Print and shaded views of the part. All mm, measured from the part's lowest x, y and z. Coordinates: 2 decimals unless noted, no trailing zeros. Loops run counter-clockwise (first coordinate to the right, second up) from the corner with the lowest first, then second, coordinate; pieces in that order, holes last. Notation, with made-up numbers: M 49.25,63.25 L 103.25,63.25 A24 cw 103.25,91.25 Z; hole C 52.25,31.5 d6. An arc over 180 degrees is marked long. Answer as CSV lines item,"result". Start each with the question number.
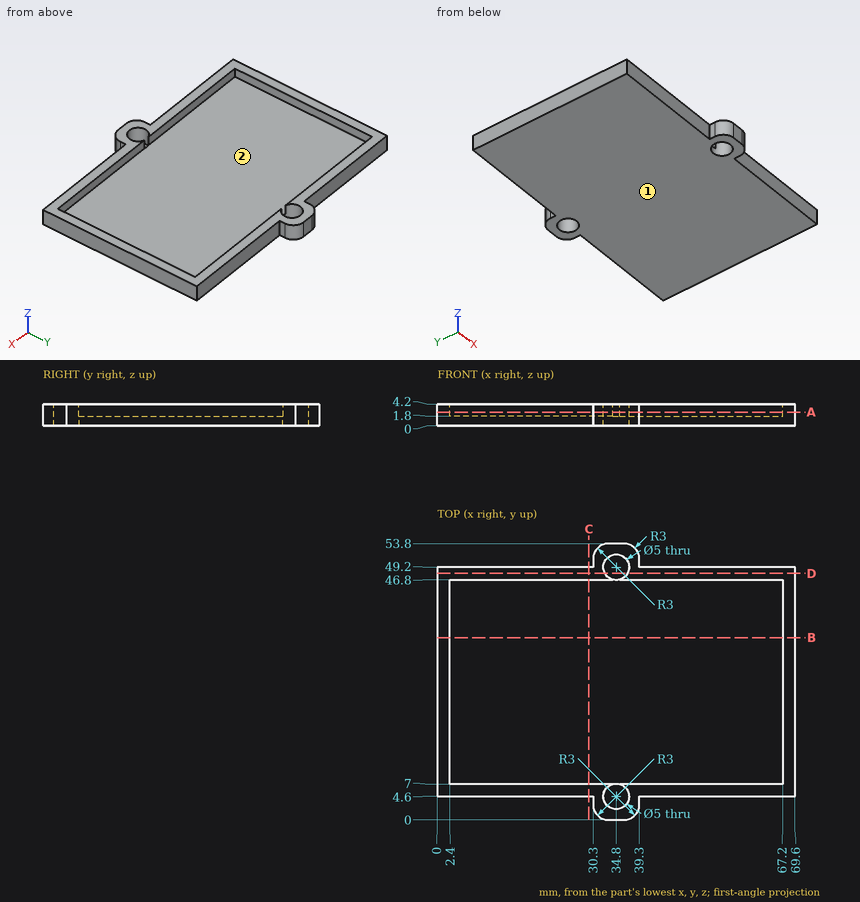
Q1. Flat gauge pins, fed straight in: P1, Ø1.3, axis at x = 22, z = 2, coming from the -Y side; P2, Ø0.8, axis at y = 50, z = 2, coming from the +X side; P3, Ø2, axis at x = 28.5, z = 0.5, coming from the +Y side. Where does each tip first touch, or does it go through?
Q2. Slice it at A-A, the plane z = 2.6. Write the cut outline in (x, y), and give its area (3 significant figures).
Q3. Slice it at C-C, the plane x = 29.5. Write the cut outline in (y, z), and give its area (3 significant figures).
Q4. Slice it at D-D, the plane y = 48. Write the cut outline in (x, z), and give its area (3 significant figures).
Q5. Slice it at B-B, the plane y = 35.5. Write the cut outline in (x, z).
Q6. Two-plate mould, pull along X, no slides. Class the marked faces 1 and 2: +X half, -X half, draft (parallel to the pull), parting line (faces both ways), or undercut.
Q7. Wall check: L1, parallel to Y at x = 34.8, z = 1.5; L2, parallel to Y at x = 43.5, z = 3.6; L3, parallel to X at y = 18.5, z = 3.1. Give the ranges that are in metal, low to high.
Solved:
1,P1,"stops at y = 4.6"
1,P2,"stops at x = 39.3"
1,P3,"stops at y = 49.2"
2,outline,"M 0,4.6 L 30.3,4.6 L 30.3,3 A3 ccw 33.3,0 L 36.3,0 A3 ccw 39.3,3 L 39.3,4.6 L 69.6,4.6 L 69.6,49.2 L 39.3,49.2 L 39.3,50.8 A3 ccw 36.3,53.8 L 33.3,53.8 A3 ccw 30.3,50.8 L 30.3,49.2 L 0,49.2 Z; hole M 2.4,7 L 34.1,7 A2.5 ccw long 35.5,7 L 67.2,7 L 67.2,46.8 L 35.5,46.8 A2.5 ccw long 34.1,46.8 L 2.4,46.8 Z"
2,area,"561 mm2"
3,outline,"M 4.6,0 L 49.2,0 L 49.2,4.2 L 46.8,4.2 L 46.8,1.8 L 7,1.8 L 7,4.2 L 4.6,4.2 Z"
3,area,"91.8 mm2"
4,outline,"M 0,0 L 32.61,0 L 32.61,4.2 L 0,4.2 Z; M 36.99,0 L 69.6,0 L 69.6,4.2 L 36.99,4.2 Z"
4,area,"274 mm2"
5,outline,"M 0,0 L 69.6,0 L 69.6,4.2 L 67.2,4.2 L 67.2,1.8 L 2.4,1.8 L 2.4,4.2 L 0,4.2 Z"
6,face 1,"draft"
6,face 2,"undercut"
7,L1,"y = 0 to 2.1, 7.1 to 46.7, 51.7 to 53.8"
7,L2,"y = 4.6 to 7, 46.8 to 49.2"
7,L3,"x = 0 to 2.4, 67.2 to 69.6"
